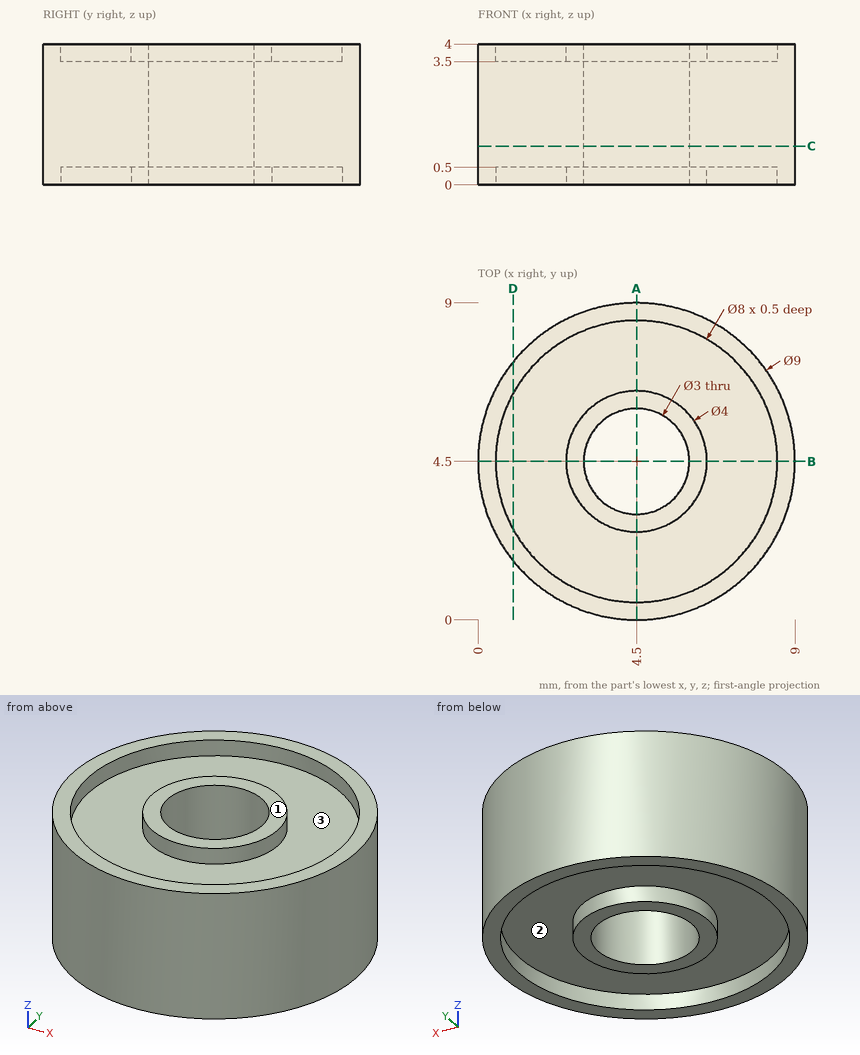
For this review, use the dimensioned drawing (mm, ordinates from the lowest corner) and the shaded views. A direction names the side the tool comes from. Give positions to 0.01 mm unless a question says otherwise; leave off trailing zeros. Order: outer loops, then holes, each group sorted by start corner. A loop starts at its lowest first (then second) coordinate and runs counter-clockwise, first axis right, second up. Notation, with made-up numbers: (2, 51.5) - (7, 51.5) arc R9 cw to (7, 55.5) - close; hole circle Ø7 at (6.5, 70.5). An arc over 180 degrees is marked (long way). Use a Markdown table: item, result. Add a question column.
(1) Add section D-D on x = 1. Give the boundary of the cut face in (y, z), then the cut area to 3 significant figures.
(2) Machinability: for the marked faces 1, 2 and 3, which of the approach directions +Z, -Z, +X, -X, +Y, -Y give a long, thin tool a straight path to every point of the face, cutting with its end or side? Answer none if there is none.
(3) Clearance check with flat-ended pins moving along their axes: P1, Ø4, axis at x = 4.5, y = 4.5, coming from the +Z side; P2, Ø1.5, axis at x = 6, z = 1.5, coming from the -Y side; P3, Ø1.5, axis at y = 5.5, z = 2, coming from the -X side; P4, Ø1, axis at y = 6, z = 3, coming from the -X side. State where each tip first meets the part, or that it passes through.
(4) Wall thickness on probe 1 along Y at (x, z) = (4.5, 0.45); probe 2 along Y at (x, z) = (4.5, 2.1); probe 3 along X at (y, z) = (6.25, 3.65): over which ranges is each line inside the solid? List them lowest first. Write a range as [from, to].
(5) Add section A-A on x = 4.5. Give the boundary of the cut face in (y, z).
(6) Add section C-C on z = 1.1. Give the boundary of the cut face in (x, y).
Report:
| question | item | result |
|---|---|---|
| 1 | outline | (1.67, 0) - (2.56, 0) - (2.56, 0.5) - (6.44, 0.5) - (6.44, 0) - (7.33, 0) - (7.33, 4) - (6.44, 4) - (6.44, 3.5) - (2.56, 3.5) - (2.56, 4) - (1.67, 4) - close |
| 1 | area | 18.8 mm² |
| 2 | face 1 | +Z, +X, -X, +Y, -Y |
| 2 | face 2 | -Z |
| 2 | face 3 | +Z |
| 3 | P1 | stops at z = 4 |
| 3 | P2 | stops at y = 0.06 |
| 3 | P3 | stops at x = 0.01 |
| 3 | P4 | stops at x = 0.11 |
| 4 | probe 1 | y = [0, 0.5], [2.5, 3], [6, 6.5], [8.5, 9] |
| 4 | probe 2 | y = [0, 3], [6, 9] |
| 4 | probe 3 | x = [0.35, 0.9], [3.53, 5.47], [8.1, 8.65] |
| 5 | outline | (0, 0) - (0.5, 0) - (0.5, 0.5) - (2.5, 0.5) - (2.5, 0) - (3, 0) - (3, 4) - (2.5, 4) - (2.5, 3.5) - (0.5, 3.5) - (0.5, 4) - (0, 4) - close; (6, 0) - (6.5, 0) - (6.5, 0.5) - (8.5, 0.5) - (8.5, 0) - (9, 0) - (9, 4) - (8.5, 4) - (8.5, 3.5) - (6.5, 3.5) - (6.5, 4) - (6, 4) - close |
| 6 | outline | circle Ø9 at (4.5, 4.5); hole circle Ø3 at (4.5, 4.5) |
